```python
from build123d import *

# Parameters (mm, degrees)
SKETCH1_W               = 50
SKETCH1_H               = 600
BOSS_EXTRUDE1_DEPTH     = 300
CUT_EXTRUDE1_DEPTH      = 428.200187266
CUT_EXTRUDE1_DEPTH_BACK = 428.200187266
SKETCH2_W               = 500
SKETCH2_H               = 550


with BuildPart() as part:
    # Sketch1 → Boss-Extrude1 (new, symmetric)
    with BuildSketch(Plane.XY):
        Rectangle(SKETCH1_W, SKETCH1_H)
    extrude(amount=BOSS_EXTRUDE1_DEPTH, both=True)

    # Sketch2 → Cut-Extrude1 (cut, two sides: drawn at the far end of the back side and taken through both)
    with BuildSketch(Plane(origin=(25, 0, 0), x_dir=(0, 0, -1), z_dir=(1, 0, 0)).offset(-CUT_EXTRUDE1_DEPTH_BACK)):
        with Locations((0, -25)):
            Rectangle(SKETCH2_W, SKETCH2_H)
    extrude(amount=CUT_EXTRUDE1_DEPTH + CUT_EXTRUDE1_DEPTH_BACK, mode=Mode.SUBTRACT)


solid = part.part
```
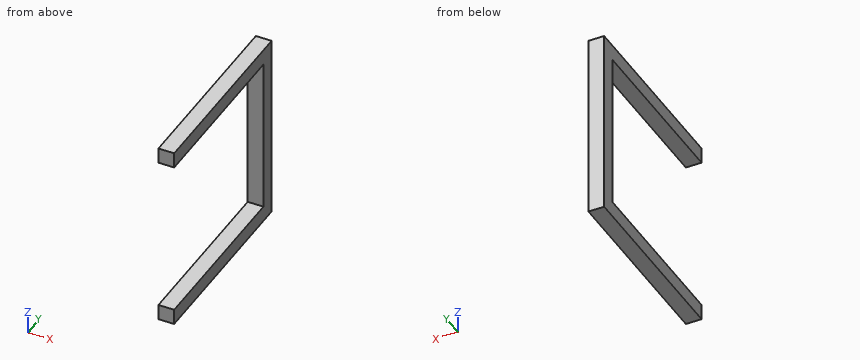
CAD build for the part. Positions are in the model's coordinates, mm. Round coordinates to 2 decimals unless told otherwise and drop trailing zeros. Order: outer loops, then holes, each group sorted by start corner. A loop starts at its lowest first (then second) coordinate and runs counter-clockwise, first axis right, second up.
Item 1: Pin check, flat tip, straight feed: pin 1 (25 mm diameter, centred on x = -6, z = 88, fed in from -Y). Stop position of the tip, or through.
Item 2: Saw through at B-B on x = 10.5. Write the cut outline in (y, z).
Item 3: Probe line 1 along Z through (x, y) = (-20, -267); line 2 along Y through (x, z) = (-16, -106.5). List the from-to ranges inside material, lowest first.
Item 4: Saw through at A-A on y = 6.5. Write the cut outline in (x, z), then the cut area to 3 significant figures.
Item 5: Saw through at C-C on z = 23. Write the cut outline in (x, y), then the cut area to 3 significant figures.
Reported:
1. pin 1: stops at y = 250
2. outline: (-300, -300) - (300, -300) - (300, 300) - (-300, 300) - (-300, 250) - (250, 250) - (250, -250) - (-300, -250) - close
3. line 1: z = -300 to -250, 250 to 300
3. line 2: y = 250 to 300
4. outline: (-25, -300) - (25, -300) - (25, -250) - (-25, -250) - close; (-25, 250) - (25, 250) - (25, 300) - (-25, 300) - close
4. area: 5,000 mm2
5. outline: (-25, 250) - (25, 250) - (25, 300) - (-25, 300) - close
5. area: 2,500 mm2
